```python
from build123d import *

# Parameters (mm, degrees)
SKETCH1_R           = 1.5
BOSS_EXTRUDE1_DEPTH = 5
SKETCH3_W           = 30
SKETCH3_H           = 25.5
BOSS_EXTRUDE2_DEPTH = 19
CUT_EXTRUDE7_DEPTH  = 26.5
FILLET10_R          = 1
FILLET11_R          = 1
CUT_EXTRUDE9_DEPTH  = 20


with BuildPart() as part:
    # Sketch1 → Boss-Extrude1 (new body)
    with BuildSketch(Plane(origin=(0, 0, 0), x_dir=(1, 0, 0), z_dir=(0, 1, 0))):
        with BuildLine():
            Line((-15.898648649, -5.337837838), (-18.648648649, -5.337837838))
            Line((-18.648648649, -5.337837838), (-18.648648649, -20.337837838))
            Line((-18.648648649, -20.337837838), (-3.648648649, -20.337837838))
            Line((-3.648648649, -20.337837838), (-3.648648649, -17.587837838))
            ThreePointArc((-3.648648649, -17.587837838), (-12.310706718, -13.999895907), (-15.898648649, -5.337837838))
        make_face()
        with Locations((-15.648648649, -17.337837838)):
            Circle(SKETCH1_R, mode=Mode.SUBTRACT)
        with BuildLine():
            ThreePointArc((8.601351351, -5.337837838), (5.013409421, -13.999895907), (-3.648648649, -17.587837838))
            Line((-3.648648649, -17.587837838), (-3.648648649, -20.337837838))
            Line((-3.648648649, -20.337837838), (11.351351351, -20.337837838))
            Line((11.351351351, -20.337837838), (11.351351351, -5.337837838))
            Line((11.351351351, -5.337837838), (8.601351351, -5.337837838))
        make_face()
        with Locations((8.351351351, -17.337837838)):
            Circle(SKETCH1_R, mode=Mode.SUBTRACT)
        with BuildLine():
            Line((-3.648648649, 9.662162162), (-3.648648649, 6.912162162))
            ThreePointArc((-3.648648649, 6.912162162), (5.013409421, 3.324220232), (8.601351351, -5.337837838))
            Line((8.601351351, -5.337837838), (11.351351351, -5.337837838))
            Line((11.351351351, -5.337837838), (11.351351351, 9.662162162))
            Line((11.351351351, 9.662162162), (-3.648648649, 9.662162162))
        make_face()
        with Locations((8.351351351, 6.662162162)):
            Circle(SKETCH1_R, mode=Mode.SUBTRACT)
        with BuildLine():
            Line((-18.648648649, 9.662162162), (-18.648648649, -5.337837838))
            Line((-18.648648649, -5.337837838), (-15.898648649, -5.337837838))
            ThreePointArc((-15.898648649, -5.337837838), (-12.310706718, 3.324220232), (-3.648648649, 6.912162162))
            Line((-3.648648649, 6.912162162), (-3.648648649, 9.662162162))
            Line((-3.648648649, 9.662162162), (-18.648648649, 9.662162162))
        make_face()
        with Locations((-15.648648649, 6.662162162)):
            Circle(SKETCH1_R, mode=Mode.SUBTRACT)
    extrude(amount=BOSS_EXTRUDE1_DEPTH)

    # Sketch3 → Boss-Extrude2 (add)
    with BuildSketch(Plane.XZ):
        with Locations((-3.648648649, 3.087837838)):
            Rectangle(SKETCH3_W, SKETCH3_H)
    extrude(amount=BOSS_EXTRUDE2_DEPTH)

    # Sketch4 → Cut-Extrude7 (cut, through all)
    with BuildSketch(Plane.XY.offset(15.837837838)):
        with BuildLine():
            ThreePointArc((7.851351351, -11.7), (4.483079335, -3.568272016), (-3.648648649, -0.2))
            Line((-3.648648649, -0.2), (-3.648648649, -19))
            Line((-3.648648649, -19), (5.237295308, -19))
            ThreePointArc((5.237295308, -19), (7.178131932, -15.57696044), (7.851351351, -11.7))
        make_face()
        with BuildLine():
            Line((-3.648648649, -19), (-3.648648649, -0.2))
            ThreePointArc((-3.648648649, -0.2), (-14.045763633, -6.78573505), (-12.534592605, -19))
            Line((-12.534592605, -19), (-3.648648649, -19))
        make_face()
        with BuildLine():
            Line((5.237295308, -19), (-3.648648649, -19))
            Line((-3.648648649, -19), (-3.648648649, -23.2))
            ThreePointArc((-3.648648649, -23.2), (1.265616301, -22.097114984), (5.237295308, -19))
        make_face()
        with BuildLine():
            Line((-3.648648649, -23.2), (-3.648648649, -19))
            Line((-3.648648649, -19), (-12.534592605, -19))
            ThreePointArc((-12.534592605, -19), (-8.562913599, -22.097114984), (-3.648648649, -23.2))
        make_face()
    extrude(amount=-CUT_EXTRUDE7_DEPTH, mode=Mode.SUBTRACT)

    # Fillet10
    fillet10_edges = [part.edges().sort_by_distance(p)[0] for p in [
        (11.351351351, 2.5, 20.337837838),
        (-18.648648649, 2.5, 20.337837838),
        (-18.648648649, 0, 18.087837838),
        (-18.648648649, -9.5, 15.837837838),
        (11.351351351, -9.5, 15.837837838),
        (11.351351351, 0, 18.087837838),
        (-3.648648649, 0, 20.337837838),
    ]]
    fillet(fillet10_edges, radius=FILLET10_R)

    # Fillet11
    fillet11_edges = [part.edges().sort_by_distance(p)[0] for p in [
        (5.237295308, -19, 3.087837838),
        (-12.534592605, -19, 3.087837838),
    ]]
    fillet(fillet11_edges, radius=FILLET11_R)

    # Sketch5 → Cut-Extrude9 (cut, through all)
    with BuildSketch(Plane(origin=(0, 0, 0), x_dir=(1, 0, 0), z_dir=(0, 1, 0))):
        with BuildLine():
            ThreePointArc((2.661066083, -15.837837838), (-3.648648649, 6.912162162), (-9.958363381, -15.837837838))
            Line((-9.958363381, -15.837837838), (2.661066083, -15.837837838))
        make_face()
    extrude(amount=-CUT_EXTRUDE9_DEPTH, mode=Mode.SUBTRACT)


solid = part.part
```
Read the model definition and answer for the solid it produces. Units are mm, in the model's axes. A direction names the side the tool comes from. Coordinates: 2 decimals unless noted, no trailing zeros. Write each loop counter-clockwise with the first axis right and the second up, starting at its lowest first coordinate (ties: lowest second). Pieces come first, ordered by that corner, then holes. Notation, with made-up numbers: (-20.5, -3) -> (-5.5, -3) arc R19 ccw to (-5.5, 24) -> close; hole circle Ø1 at (7.25, 33). An arc over 180 degrees is marked (long way). Answer as a JSON object with one key per item and string values.
Q1. Flat-ended cylindrical pins translate along their axes: pin 1 Ø1.8 at (x, z) = (-15.65, 17.34) entering from +Y; pin 2 Ø1 at (x, z) = (3, 18) entering from -Y; pin 3 Ø1.5 at (x, y) = (7, -13.5) entering from +Z; pin 4 Ø2.5 at (x, z) = (8.35, -6.66) entering from +Y. Find the tip coordinate at first contact, or state that the pin passes through.
The answers:
{"pin 1": "passes through", "pin 2": "stops at y = 0", "pin 3": "stops at z = 15.84", "pin 4": "stops at y = 0"}
Q2. Determine the mould class of faces 6 (the cylindrical face through (-13.585, -18.511, 13.972)), 7 (the flat face through (8, 0, -7)), 8 (the cylindrical face through (-14.26, 2.46, -6.09)) for opening direction Y: pulls with the +Y half, pulls with the -Y half, needs draft (parallel to the pull), parting line crosses it, or undercut.
The answers:
{"face 6": "undercut", "face 7": "pulls with the +Y half", "face 8": "needs draft"}
Q3. The part is cut by section D-D on y = 2.75. Give the vertices of the cut face in (x, z), then the cut area to 3 significant figures.
The answers:
{"outline": "(-18.65, -9.66) -> (11.35, -9.66) -> (11.35, 19.34) arc R1 ccw to (10.35, 20.34) -> (-17.65, 20.34) arc R1 ccw to (-18.65, 19.34) -> close; hole circle Ø3 at (-15.65, -6.66); hole circle Ø3 at (-15.65, 17.34); hole circle Ø24.5 at (-3.65, 5.34); hole circle Ø3 at (8.35, -6.66); hole circle Ø3 at (8.35, 17.34)", "area": "400 mm2"}
Q4. The part is cut by section A-A on y = -16.25. Give the vertices of the cut face in (x, z), then the cut area to 3 significant figures.
The answers:
{"outline": "(-18.65, -9.66) -> (-14.21, -9.66) -> (-14.21, -0.87) arc R12.25 cw to (-14.21, 11.54) -> (-14.21, 15.84) -> (-17.65, 15.84) arc R1 ccw to (-18.65, 14.84) -> close; (6.91, -9.66) -> (11.35, -9.66) -> (11.35, 14.84) arc R1 ccw to (10.35, 15.84) -> (6.91, 15.84) -> (6.91, 11.54) arc R12.25 cw to (6.91, -0.87) -> close", "area": "198 mm2"}
Q5. Consider line 1 (Z direction, x = -16.5, y = -9.75); line 2 (Z direction, x = -14.5, y = 2.25); line 3 (X direction, y = 0.75, z = 5). Determine where each line is inside the solid, lowest interval first. Write a range as [from, to].
The answers:
{"line 1": "z = [-9.66, 15.84]", "line 2": "z = [-9.66, -7.63], [-5.7, -0.35], [11.02, 16.37], [18.3, 20.34]", "line 3": "x = [-18.65, -15.89], [8.6, 11.35]"}
Q6. The part is cut by section C-C on z = -3. Give the vertices of the cut face in (x, y).
The answers:
{"outline": "(-18.65, -19) -> (-14.44, -19) arc R1 ccw to (-13.58, -17.5) arc R11.5 cw to (-12.62, -4.51) -> (-12.62, 5) -> (-18.65, 5) -> close; (5.33, -4.51) arc R11.5 cw to (6.28, -17.5) arc R1 ccw to (7.15, -19) -> (11.35, -19) -> (11.35, 5) -> (5.33, 5) -> close"}
Q7. The part is cut by section B-B on x = -8. Give the vertices of the cut face in (y, z).
The answers:
{"outline": "(-1.06, -9.66) -> (5, -9.66) -> (5, -6.11) -> (-1.06, -6.11) -> close; (0, 16.79) -> (5, 16.79) -> (5, 20.34) -> (1, 20.34) arc R1 ccw to (0, 19.34) -> close"}
Q8. A tool of negligible diameter and unlimited length cuts with its end or side. For faces 1 (the cylindrical face through (-18.4, -9.1, 15.5)), 2 (the flat face through (-16, -7, 15.838)), 3 (the cylindrical face through (11.051, 0.285, 17.556)), 4 (the flat face through (-17, -19, 3)), 5 (the cylindrical face through (6.288, -18.511, -5.121)), from which of +Z, -Z, +X, -X, +Y, -Y can it reach the whole face along a straight path? Write none if from no direction.
The answers:
{"face 1": "+Z, -X, -Y", "face 2": "+Z, +X, -X, -Y", "face 3": "+Z, +X, -Y", "face 4": "+Z, -Z, +X, -X, -Y", "face 5": "+Z, -Z"}
